Verification items for the finished model (mm, model axes). Round coordinates to 2 decimals unless told otherwise and drop trailing zeros. Loops run counter-clockwise (first coordinate to the right, second up) from the corner with the lowest first, then second, coordinate; pieces in that order, holes last. Notation, with made-up numbers: (-24, 29.5) -> (34, 29.5) arc R14 cw to (34, 55.5) -> close; hole circle Ø4 at (-23, -23). An arc over 180 degrees is marked (long way). Write item = value, one per line. Start each with the question number.
```python
from build123d import *

# Parameters (mm, degrees)
SKETCH1_W               = 25.4
SKETCH1_H               = 12.7
BOSS_EXTRUDE1_DEPTH     = 127
SKETCH4_W               = 22.225
SKETCH4_H               = 9.525
CUT_EXTRUDE1_DEPTH      = 128
SKETCH5_R               = 1.7526
CUT_EXTRUDE2_DEPTH      = 1
CUT_EXTRUDE2_DEPTH_BACK = 13.7
SKETCH6_R               = 1.5
CUT_EXTRUDE3_DEPTH      = 1
CUT_EXTRUDE3_DEPTH_BACK = 13.7
SKETCH7_W               = 25.4
SKETCH7_H               = 12.7
SKETCH7_W_2             = 22.225
SKETCH7_H_2             = 9.525
BOSS_EXTRUDE2_DEPTH     = 25.4


with BuildPart() as part:
    # Sketch1 → Boss-Extrude1 (new body)
    with BuildSketch(Plane.XY):
        Rectangle(SKETCH1_W, SKETCH1_H)
    extrude(amount=BOSS_EXTRUDE1_DEPTH)

    # Sketch4 → Cut-Extrude1 (cut, through all)
    with BuildSketch(Plane(origin=(0, 0, 0), x_dir=(-1, 0, 0), z_dir=(0, 0, -1))):
        Rectangle(SKETCH4_W, SKETCH4_H)
    extrude(amount=-CUT_EXTRUDE1_DEPTH, mode=Mode.SUBTRACT)

    # Sketch5 → Cut-Extrude2 (cut, two sides)
    with BuildSketch(Plane(origin=(0, 6.35, 0), x_dir=(1, 0, 0), z_dir=(0, 1, 0))) as cut_extrude2_sk:
        with Locations((-5.588, -123.825)):
            Circle(SKETCH5_R)
        with Locations((5.5372, -123.825)):
            Circle(SKETCH5_R)
    extrude(amount=CUT_EXTRUDE2_DEPTH, mode=Mode.SUBTRACT)
    extrude(cut_extrude2_sk.sketch, amount=-CUT_EXTRUDE2_DEPTH_BACK, mode=Mode.SUBTRACT)

    # Sketch6 → Cut-Extrude3 (cut, two sides)
    with BuildSketch(Plane(origin=(0, -6.35, 0), x_dir=(-1, 0, 0), z_dir=(0, -1, 0))) as cut_extrude3_sk:
        with Locations((8, -11.05)):
            Circle(SKETCH6_R)
        with Locations((-8, -11.05)):
            Circle(SKETCH6_R)
        with Locations((0, -3.05)):
            Circle(SKETCH6_R)
        with Locations((0, -19.05)):
            Circle(SKETCH6_R)
    extrude(amount=CUT_EXTRUDE3_DEPTH, mode=Mode.SUBTRACT)
    extrude(cut_extrude3_sk.sketch, amount=-CUT_EXTRUDE3_DEPTH_BACK, mode=Mode.SUBTRACT)

    # Sketch7 → Boss-Extrude2 (add)
    with BuildSketch(Plane(origin=(0, 0, 0), x_dir=(-1, 0, 0), z_dir=(0, 0, -1))):
        Rectangle(SKETCH7_W, SKETCH7_H)
        Rectangle(SKETCH7_W_2, SKETCH7_H_2, mode=Mode.SUBTRACT)
    extrude(amount=BOSS_EXTRUDE2_DEPTH)


solid = part.part
```
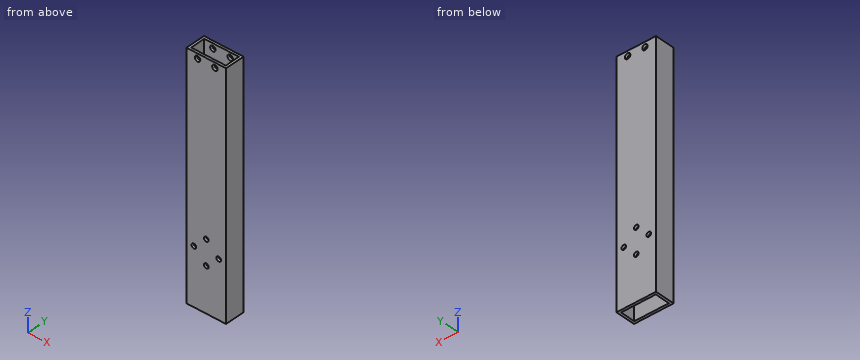
(1) Scan lines: line 1 (Z direction, x = 0, y = -5.25); line 2 (X direction, y = 5.95, z = 11.05); line 3 (Y direction, x = 7.75, z = 71). Record each from-to range of solid material in increasing order. Write a range as [from, to].
(2) Depth check by flat-ended pin: pin 1 Ø5 at (x, z) = (0, 19.05) entering from +Y. Enter the tip coordinate at first touch or a pass-through.
(3) Section check B-B on z = 11.05. Enter the section's corners in (x, y), then the cut area to 3 significant figures.
(4) Section check C-C on z = 100.5. Enter the section's corners in (x, y), then the cut area to 3 significant figures.
(5) Section check A-A on y = -1.25. Enter the section's corners in (x, z), then the cut area to 3 significant figures.
Computed values:
q1.line_1 = [-25.4, 1.55], [4.55, 17.55], [20.55, 127]
q1.line_2 = [-12.7, -9.5], [-6.5, 6.5], [9.5, 12.7]
q1.line_3 = [-6.35, -4.76], [4.76, 6.35]
q2.pin_1 = 6.35
q3.outline = (-12.7, -6.35) -> (-9.5, -6.35) -> (-9.5, -4.76) -> (-11.11, -4.76) -> (-11.11, 4.76) -> (-9.5, 4.76) -> (-9.5, 6.35) -> (-12.7, 6.35) -> close; (-6.5, -6.35) -> (6.5, -6.35) -> (6.5, -4.76) -> (-6.5, -4.76) -> close; (-6.5, 4.76) -> (6.5, 4.76) -> (6.5, 6.35) -> (-6.5, 6.35) -> close; (9.5, -6.35) -> (12.7, -6.35) -> (12.7, 6.35) -> (9.5, 6.35) -> (9.5, 4.76) -> (11.11, 4.76) -> (11.11, -4.76) -> (9.5, -4.76) -> close
q3.area = 91.8 mm²
q4.outline = (-12.7, -6.35) -> (12.7, -6.35) -> (12.7, 6.35) -> (-12.7, 6.35) -> close; hole (-11.11, -4.76) -> (11.11, -4.76) -> (11.11, 4.76) -> (-11.11, 4.76) -> close
q4.area = 111 mm²
q5.outline = (-12.7, -25.4) -> (-11.11, -25.4) -> (-11.11, 127) -> (-12.7, 127) -> close; (11.11, -25.4) -> (12.7, -25.4) -> (12.7, 127) -> (11.11, 127) -> close
q5.area = 484 mm²
